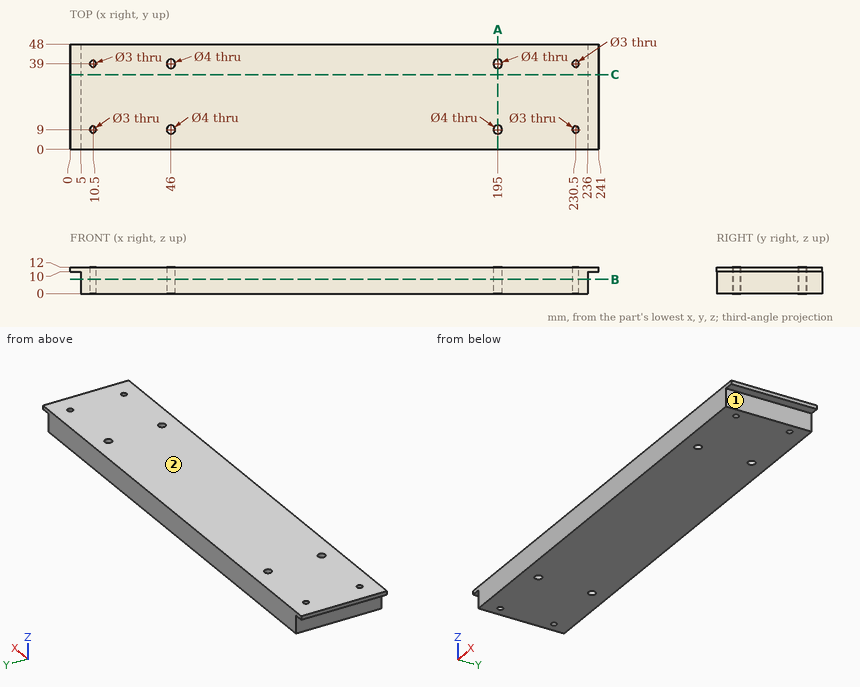
Geometry: see drawing. Coordinates: mm, zero at the bounding-box minimum. A direction names the side the tool comes from. Round coordinates to 2 decimals unless told otherwise and drop trailing zeros. Loops run counter-clockwise (first coordinate to the right, second up) from the corner with the lowest first, then second, coordinate; pieces in that order, holes last. Notation, with made-up numbers: (17.5, 41.25) -> (75.5, 41.25) arc R26 ccw to (75.5, 75.25) -> close; hole circle Ø7 at (-28.75, -4). An arc over 180 degrees is marked (long way). Write each question's results on one line, items separated by ' | '.
Item 1: Pin query (flat end, axial travel): pin 1 Ø5 at (y, z) = (13.5, 4.5) entering from -X; pin 2 Ø1.5 at (x, y) = (2, 13) entering from -Z; pin 3 Ø5 at (y, z) = (25.5, 2) entering from +X; pin 4 Ø2.5 at (x, y) = (10.5, 39) entering from -Z. Return the tip coordinate at first contact, or that it passes through.
Answers below:
pin 1: stops at x = 5 | pin 2: stops at z = 10 | pin 3: stops at x = 236 | pin 4: passes through
Item 2: Line query: probe 1 along Y at (x, z) = (46, 8.5); probe 2 along Y at (x, z) = (10.5, 3.25); probe 3 along X at (y, z) = (8, 7). Output: solid intervals per line, ascending. Write a range as [from, to].
Answers below:
probe 1: y = [0, 7], [11, 37], [41, 48] | probe 2: y = [0, 7.5], [10.5, 37.5], [40.5, 48] | probe 3: x = [5, 9.38], [11.62, 44.27], [47.73, 193.27], [196.73, 229.38], [231.62, 236]
Item 3: Set-up query: the marked faces 1 and 2. Return all of +Z, -Z, +X, -X, +Y, -Y with unobstructed straight access to the full face (end or side cutting, diameter ignored); none if empty.
Answers below:
face 1: -Z, +X, +Y, -Y | face 2: +Z, +X, -X, +Y, -Y
Item 4: Cut plane A-A on x = 195. Return the cut outline in (y, z).
Answers below:
outline: (0, 0) -> (7, 0) -> (7, 12) -> (0, 12) -> close; (11, 0) -> (37, 0) -> (37, 12) -> (11, 12) -> close; (41, 0) -> (48, 0) -> (48, 12) -> (41, 12) -> close
Item 5: Cut plane C-C on y = 34. Return the cut outline in (x, z).
Answers below:
outline: (0, 10) -> (5, 10) -> (5, 0) -> (236, 0) -> (236, 10) -> (241, 10) -> (241, 12) -> (0, 12) -> close
Item 6: Cut plane B-B on z = 6.5. State how many separate pieces and enclosed holes the cut face has, and give its area (3 significant figures).
Answers below:
separate pieces: 1 | enclosed holes: 8 | area: 11,000 mm²
